Source: three-view drawing plus pictorial views. Frame: mm from the lowest corner of the part. A direction names the side the tool comes from. Give positions to 0.01 mm unless a question says otherwise; leave off trailing zeros. Order: outer loops, then holes, each group sorted by start corner. A loop starts at its lowest first (then second) coordinate and runs counter-clockwise, first axis right, second up. Notation, with made-up numbers: (25.25, 7) -> (82.25, 7) arc R11 cw to (82.25, 18) -> close; hole circle Ø1 at (36.25, -4.5). An arc over 180 degrees is marked (long way). Answer in a Markdown table with one row per item.
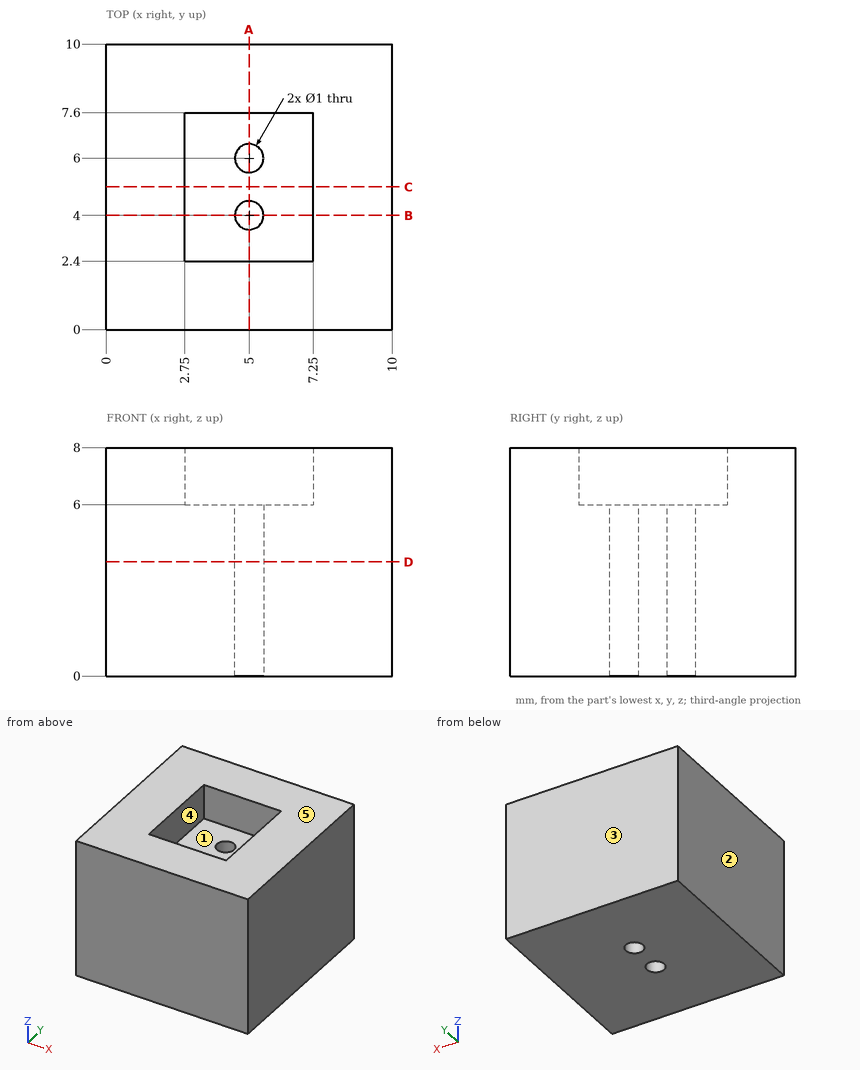
(1) Access query for the marked faces 4 and 5. Directions: +Z, -Z, +X, -X, +Y, -Y. A direction counts if a zero-diameter tool reaches every point of the face in a straight line with its end or side. Return the directions, or none.
A:
| item | result |
|---|---|
| face 4 | +Z |
| face 5 | +Z, +X, -X, +Y, -Y |
(2) Ray query, probe 1 along Y at (x, z) = (5, 1.55); probe 2 along Y at (x, z) = (4.25, 7.75); probe 3 along Z at (x, y) = (6.5, 3.5). Return the intervals inside material, ascending.
A:
| item | result |
|---|---|
| probe 1 | y = 0 to 3.5, 4.5 to 5.5, 6.5 to 10 |
| probe 2 | y = 0 to 2.4, 7.6 to 10 |
| probe 3 | z = 0 to 6 |
(3) Section query B-B (y = 4). Return the cut outline in (x, z).
A:
| item | result |
|---|---|
| outline | (0, 0) -> (4.5, 0) -> (4.5, 6) -> (2.75, 6) -> (2.75, 8) -> (0, 8) -> close; (5.5, 0) -> (10, 0) -> (10, 8) -> (7.25, 8) -> (7.25, 6) -> (5.5, 6) -> close |
(4) Section query C-C (y = 5). Return the cut outline in (x, z).
A:
| item | result |
|---|---|
| outline | (0, 0) -> (10, 0) -> (10, 8) -> (7.25, 8) -> (7.25, 6) -> (2.75, 6) -> (2.75, 8) -> (0, 8) -> close |
(5) Pull-direction query (Y, two-part tool) for the marked faces 1, 2 and 3; classes: +Y half, -Y half, draft (parallel to the pull), parting line (faces both ways), or undercut.
A:
| item | result |
|---|---|
| face 1 | undercut |
| face 2 | draft |
| face 3 | +Y half |
(6) Section query D-D (z = 4). Return the cut outline in (x, y), plus the area to 3 significant figures.
A:
| item | result |
|---|---|
| outline | (0, 0) -> (10, 0) -> (10, 10) -> (0, 10) -> close; hole circle Ø1 at (5, 4); hole circle Ø1 at (5, 6) |
| area | 98.4 mm^2 |
(7) Section query A-A (x = 5). Return the cut outline in (y, z).
A:
| item | result |
|---|---|
| outline | (0, 0) -> (3.5, 0) -> (3.5, 6) -> (2.4, 6) -> (2.4, 8) -> (0, 8) -> close; (4.5, 0) -> (5.5, 0) -> (5.5, 6) -> (4.5, 6) -> close; (6.5, 0) -> (10, 0) -> (10, 8) -> (7.6, 8) -> (7.6, 6) -> (6.5, 6) -> close |
(8) First-contact query: pin 1 Ø2 at (x, y) = (5, 5) entering from +Z. Flat tip, straight axial feed; report the tip coordinate or a pass-through.
A:
| item | result |
|---|---|
| pin 1 | stops at z = 6 |
